The model under review builds one solid part; all positions refer to its coordinate system, in mm. A direction names the side the tool comes from. Round coordinates to 2 decimals unless told otherwise and drop trailing zeros. Order: outer loops, then holes, each group sorted by start corner. A loop starts at its lowest first (then second) coordinate and runs counter-clockwise, first axis right, second up. Notation, with made-up numbers: M -22,-18.5 L -16,-18.5 A26 cw -16,15.5 Z; hole C 50,23.5 d1. An arc over 180 degrees is marked long. Answer as CSV lines item,"result". Start each with the question number.
from build123d import *

# Parameters (mm, degrees)
F1_DEPTH = 5
F3_DEPTH = 4


with BuildPart() as f1:
    # F0 (on Top) → F1 (new body)
    with BuildSketch(Plane.XY):
        Polygon((0, -35), (0, 0), (-9.510925, 12.472135), (-26.420884, 21.336073), (-45.579116, 21.336073), (-64.596242, 10.46882), (-75.796338, -13.468692), (-71.267544, -15.587665), (-60.739219, 6.914099), (-44.251259, 16.33607), (-27.65191, 16.33607), (-12.814397, 8.558477), (-5.000003, -1.688916), (-5.000003, -33.450294), (-10.299125, -41.177687), (-19.113462, -48.230996), (-15.989488, -52.134945), (-6.595456, -44.617758), align=None)
    extrude(amount=F1_DEPTH)

    # F2 (on face) → F3 (cut)
    with BuildSketch(Plane.YZ):
        Polygon((-4.5, 0), (-4.5, 2.5), (-4.5, 5), (-30.5, 5), (-30.5, 2.5), (-30.5, 0), align=None)
    extrude(amount=-F3_DEPTH, mode=Mode.SUBTRACT)


with BuildPart() as f4_1:
    # F4: copy of F1
    add(f1.part)


solid = f4_1.part
Item 1: The part is to be moulded in two halves that separate along X. For faces 5 (the flat face through (-70.118, -1.332, 2.465)), 6 (the flat face through (-5, -17, 2)), 7 (the flat face through (0, -2, 2)), say which applies: +X half, -X half, draft (parallel to the pull), parting line (faces both ways), or undercut.
Item 2: Consider section A-A (z = 2.25). State the section outline as (x, y) points, and give its area (3 significant figures).
Item 3: Wall thickness on probe 1 along X at (y, z) = (-20, 3.8); probe 2 along Y at (x, z) = (-8.5, 1.7); probe 3 along X at (y, z) = (11, 4.55): over which ranges is each line inside the solid? List them lowest first. Write a range as [from, to].
Item 4: Tool access review of faces 1 (the flat face through (-20.337, 12.502, 2.465)), 2 (the flat face through (-4, -18, 3)), 3 (the flat face through (-66.077, -4.494, 2.465)), 4 (the flat face through (-14.64, -44.65, 2.46)): name each direction out of +Z, -Z, +X, -X, +Y, -Y from which nothing blocks a thin tool from reaching the whole face with its end or side.
Item 5: Consider section D-D (y = -20.5). State the section outline as (x, z) points, and give its area (3 significant figures).
Item 6: Consider section C-C (x = -42). State the section outline as (y, z) points.
Item 7: For pin 1 (1.5 mm diameter, centred on x = -8.5, z = 4, fed in from +Y); pin 2 (1.5 mm diameter, centred on y = -14, z = 2.5, fed in from +X); pin 3 (1.2 mm diameter, centred on x = -2.5, z = 2.5, fed in from -Y), all flat-tipped, find the tip position at first contact; note any pin that passes through.
Item 8: Consider section B-B (y = 3). State the section outline as (x, z) points, and give its area (3 significant figures).
Reported:
1,face 5,"-X half"
1,face 6,"undercut"
1,face 7,"+X half"
2,outline,"M -75.8,-13.47 L -71.27,-15.59 L -60.74,6.91 L -44.25,16.34 L -27.65,16.34 L -12.81,8.56 L -5,-1.69 L -5,-33.45 L -10.3,-41.18 L -19.11,-48.23 L -15.99,-52.13 L -6.6,-44.62 L 0,-35 L 0,-30.5 L -4,-30.5 L -4,-4.5 L 0,-4.5 L 0,0 L -9.51,12.47 L -26.42,21.34 L -45.58,21.34 L -64.6,10.47 Z"
2,area,"655 mm²"
3,probe 1,"x = [-5, -4]"
3,probe 2,"y = [-46.14, -38.55], [2.9, 11.15]"
3,probe 3,"x = [-63.67, -53.59], [-17.47, -8.39]"
4,face 1,"+Z, -Z"
4,face 2,"+Z, -Z, +X"
4,face 3,"+Z, -Z, -Y"
4,face 4,"+Z, -Z, -X"
5,outline,"M -5,0 L -4,0 L -4,5 L -5,5 Z"
5,area,"5.00 mm²"
6,outline,"M 16.34,0 L 21.34,0 L 21.34,5 L 16.34,5 Z"
7,pin 1,"stops at y = 12.13"
7,pin 2,"stops at x = -4"
7,pin 3,"stops at y = -39.52"
8,outline,"M -68.09,0 L -62.57,0 L -62.57,5 L -68.09,5 Z; M -8.58,0 L -2.29,0 L -2.29,5 L -8.58,5 Z"
8,area,"59.0 mm²"
